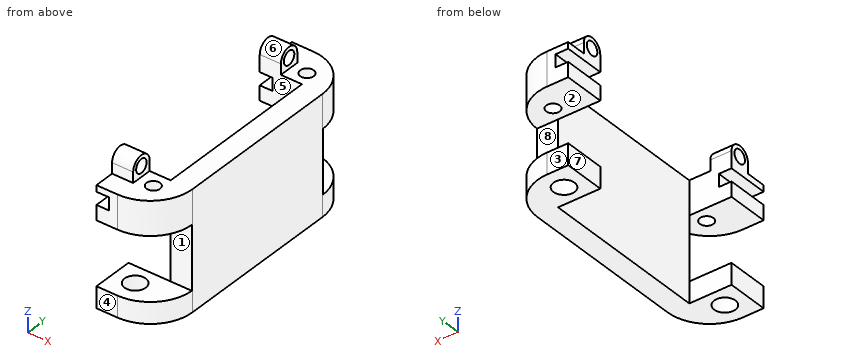
from build123d import *
from build123d.topology import SkipClean

# Parameters (mm, degrees)
BOSS_EXTRUDE1_DEPTH = 8
SKETCH2_W           = 20
SKETCH2_H           = 40
BOSS_EXTRUDE2_DEPTH = 5
SKETCH3_W           = 5
SKETCH3_H           = 5
BOSS_EXTRUDE3_DEPTH = 5
FILLET2_RADIUS      = 2.5
FILLET2_LENGTH      = 5
FILLET3_RADIUS      = 2.5
FILLET3_LENGTH      = 5
SKETCH6_R           = 1.6
CUT_EXTRUDE3_DEPTH  = 34.541019662
BOSS_EXTRUDE4_DEPTH = 5
BOSS_EXTRUDE5_DEPTH = 5
SKETCH11_W          = 15
SKETCH11_H          = 4.771622141
BOSS_EXTRUDE6_DEPTH = 8
FILLET4_R           = 10
FILLET5_START       = -21
FILLET5_DEPTH       = 30
SKETCH12_R          = 1.6
CUT_EXTRUDE4_DEPTH  = 10
SKETCH15_W          = 6
SKETCH15_H          = 3
CUT_EXTRUDE7_DEPTH  = 20
SKETCH17_W          = 6
SKETCH17_H          = 3
CUT_EXTRUDE8_DEPTH  = 20


with BuildPart() as part:
    # Sketch1 → Boss-Extrude1 (new body)
    with BuildSketch(Plane.XY):
        Polygon((-5, 25), (10, 25), (10, -25), (-5, -25), (-5, -20), (5, -20), (5, 20), (-5, 20), align=None)
    extrude(amount=BOSS_EXTRUDE1_DEPTH)

    # Sketch2 → Boss-Extrude2 (add)
    with BuildSketch(Plane(origin=(10, 0, 0), x_dir=(0, 0, -1), z_dir=(1, 0, 0))):
        with Locations((10, 0)):
            Rectangle(SKETCH2_W, SKETCH2_H)
    extrude(amount=-BOSS_EXTRUDE2_DEPTH)

    # Sketch3 → Boss-Extrude3 (add)
    with BuildSketch(Plane.XY.offset(8)):
        with Locations((-2.5, 22.5)):
            Rectangle(SKETCH3_W, SKETCH3_H)
        with Locations((-2.5, -22.5)):
            Rectangle(SKETCH3_W, SKETCH3_H)
    extrude(amount=BOSS_EXTRUDE3_DEPTH)

    # Fillet2: full round fillet: the end face becomes a half cylinder, R = half its width
    fillet2_face = Plane((-2.5, 22.5, 13), x_dir=(1, 0, 0), z_dir=(0, 0, 1))  # on the end face: x along it, z out of the body
    fillet2_slab = fillet2_face.offset(-FILLET2_RADIUS / 2) * Box(FILLET2_LENGTH, 2 * FILLET2_RADIUS, FILLET2_RADIUS, mode=Mode.PRIVATE)  # the body's end, R deep
    fillet2_round = Plane((-2.5, 22.5, 10.5), x_dir=(0, 0, 1), z_dir=(1, 0, 0)) * Cylinder(FILLET2_RADIUS, FILLET2_LENGTH, mode=Mode.PRIVATE)  # its axis R under the face
    add(fillet2_slab - fillet2_round, mode=Mode.SUBTRACT)

    # Fillet3: full round fillet: the end face becomes a half cylinder, R = half its width
    fillet3_face = Plane((-2.5, -22.5, 13), x_dir=(1, 0, 0), z_dir=(0, 0, 1))  # on the end face: x along it, z out of the body
    fillet3_slab = fillet3_face.offset(-FILLET3_RADIUS / 2) * Box(FILLET3_LENGTH, 2 * FILLET3_RADIUS, FILLET3_RADIUS, mode=Mode.PRIVATE)  # the body's end, R deep
    fillet3_round = Plane((-2.5, -22.5, 10.5), x_dir=(0, 0, 1), z_dir=(1, 0, 0)) * Cylinder(FILLET3_RADIUS, FILLET3_LENGTH, mode=Mode.PRIVATE)  # its axis R under the face
    add(fillet3_slab - fillet3_round, mode=Mode.SUBTRACT)

    # Sketch6 → Cut-Extrude3 (cut, through all)
    with BuildSketch(Plane(origin=(0, 0, 0), x_dir=(0, 0, -1), z_dir=(1, 0, 0))):
        with Locations((-10.5, 22.5)):
            Circle(SKETCH6_R)
        with Locations((-10.5, -22.5)):
            Circle(SKETCH6_R)
    extrude(amount=-CUT_EXTRUDE3_DEPTH, mode=Mode.SUBTRACT)

    # Sketch7 → Boss-Extrude4 (add)
    with BuildSketch(Plane(origin=(0, 0, -20), x_dir=(-1, 0, 0), z_dir=(0, 0, -1))):
        with BuildLine():
            Line((5, 27.3), (5, 20))
            Line((5, 20), (-5, 20))
            Line((-5, 20), (-10, 20))
            Line((-10, 20), (-10, 27.3))
            Line((-10, 27.3), (-1.58, 27.3))
            Line((-1.58, 27.3), (-1.58, 26.5))
            ThreePointArc((-1.58, 26.5), (-0.08, 22), (1.42, 26.5))
            Line((1.42, 26.5), (1.42, 27.3))
            Line((1.42, 27.3), (5, 27.3))
        make_face()
    boss_extrude4 = extrude(amount=-BOSS_EXTRUDE4_DEPTH)

    # Mirror3: Boss-Extrude4 across plane
    add(boss_extrude4.mirror(Plane.ZX))

    # Sketch10 → Boss-Extrude5 (add)
    with SkipClean():  # the faces are left unmerged after this step: merging them gives an invalid solid
        with BuildSketch(Plane(origin=(0, 0, -20), x_dir=(-1, 0, 0), z_dir=(0, 0, -1))):
            with BuildLine():
                Line((5, 29.771622141), (-10, 29.771622141))
                Line((-10, 29.771622141), (-10, 27.3))
                Line((-10, 27.3), (-1.58, 27.3))
                Line((-1.58, 27.3), (-1.58, 26.5))
                ThreePointArc((-1.58, 26.5), (-0.08, 27), (1.42, 26.5))
                Line((1.42, 26.5), (1.42, 27.3))
                Line((1.42, 27.3), (5, 27.3))
                Line((5, 27.3), (5, 29.771622141))
            make_face()
        boss_extrude5 = extrude(amount=-BOSS_EXTRUDE5_DEPTH)

    # Mirror4: Boss-Extrude5 across plane
    with SkipClean():  # the faces are left unmerged after this step: merging them gives an invalid solid
        add(boss_extrude5.mirror(Plane.ZX))

    # Sketch11 → Boss-Extrude6 (add)
    with SkipClean():  # the faces are left unmerged after this step: merging them gives an invalid solid
        with BuildSketch(Plane.XY.offset(8)):
            with Locations((2.5, 27.385811071)):
                Rectangle(SKETCH11_W, SKETCH11_H)
            with Locations((2.5, -27.385811071)):
                Rectangle(SKETCH11_W, SKETCH11_H)
        extrude(amount=-BOSS_EXTRUDE6_DEPTH)

    # Fillet4
    # the kernel refuses this fillet: 10 mm, written as the material it takes off along each edge
    with BuildSketch(Plane(origin=(10, 29.771622141, 33), x_dir=(0, -1, 0), z_dir=(0, 0, -1))) as fillet4_piece_1:
        with BuildLine():
            CenterArc((FILLET4_R, FILLET4_R), FILLET4_R, 180, 90)
            Line((0, FILLET4_R), (0, 0))
            Line((0, 0), (FILLET4_R, 0))
        make_face()
    extrude(amount=58, mode=Mode.SUBTRACT)

    # Fillet5: read off the stored shape, not the designer's step
    # Fillet5 outline → Fillet5 (cut)
    with BuildSketch(Plane.XY.offset(FILLET5_START)):
        with BuildLine():
            Line((10, -29.771622141), (10, -19.771622141))
            ThreePointArc((10, -19.771622141), (7.071067812, -26.842689953), (0, -29.771622141))
            Line((0, -29.771622141), (10, -29.771622141))
        make_face()
    extrude(amount=FILLET5_DEPTH, mode=Mode.SUBTRACT)

    # Sketch12 → Cut-Extrude4 (cut)
    with BuildSketch(Plane.XY.offset(8)):
        with Locations((3.535533906, 23.421344977)):
            Circle(SKETCH12_R)
        with Locations((3.535533906, -23.421344977)):
            Circle(SKETCH12_R)
    extrude(amount=-CUT_EXTRUDE4_DEPTH, mode=Mode.SUBTRACT)

    # Sketch15 → Cut-Extrude7 (cut)
    with BuildSketch(Plane.XZ.offset(29.771622141)):
        with Locations((-5, 5)):
            Rectangle(SKETCH15_W, SKETCH15_H)
    extrude(amount=-CUT_EXTRUDE7_DEPTH, mode=Mode.SUBTRACT)

    # Sketch17 → Cut-Extrude8 (cut)
    with BuildSketch(Plane(origin=(0, 29.771622141, 0), x_dir=(1, 0, 0), z_dir=(0, 1, 0))):
        with Locations((-5, -5)):
            Rectangle(SKETCH17_W, SKETCH17_H)
    extrude(amount=-CUT_EXTRUDE8_DEPTH, mode=Mode.SUBTRACT)


solid = part.part
CAD build for the part. Positions are in the model's coordinates, mm. Face numbers are marked on the shaded views. A direction names the side the tool comes from. Round coordinates to 2 decimals unless told otherwise and drop trailing zeros. Write each loop counter-clockwise with the first axis right and the second up, starting at its lowest first coordinate (ties: lowest second). Pieces come first, ordered by that corner, then holes. Notation, with made-up numbers: M 11,-33 L 56,-33 A16 cw 56,-26 Z; hole C -2,89 d5. An arc over 180 degrees is marked long. Put each result on its own line as item: value. Start each with the question number.
1) Pin check, flat tips, straight feed: pin 1 Ø2.5 at (x, y) = (3.54, 23.42) entering from +Z; pin 2 Ø5.5 at (y, z) = (-22.5, 11) entering from +X; pin 3 Ø1.5 at (x, z) = (7.5, -11) entering from +Y. Stop position of each tip, or through.
2) Saw through at A-A, the plane x = -3.75. Count the separate pieces of the cut face and the enclosed holes in it, and give its area (3 significant figures).
3) Saw through at C-C, the plane z = 4.5. Write the cut outline in (x, y).
4) Saw through at D-D, the plane z = -11.5. Write the cut outline in (x, y).
5) Saw through at B-B, the plane x = 0.75. Write the cut outline in (y, z).
6) Drill centre lines: probe 1 along Y at (x, z) = (0.08, -18.1); probe 2 along Z at (x, y) = (8.5, -22); probe 3 along Y at (x, z) = (-3.65, 10.5). Where is each one in solid material? Low to high. Write a range as [from, to].
7) 3-axis set-ups, long thin cutter, end or side, ignore diameter. For the marked faces 1, 2, 3, 4 and 5: which of +Z, -Z, +X, -X, +Y, -Y reach the whole face in a straight line?
8) Pull direction Z, two halves, no side cores. Call the marked faces 6, 7 and 8: pulls with the +Z half, pulls with the -Z half, needs draft (parallel to the pull), parting line crosses it, or undercut.
Resolved:
1. pin 1: z = -15
1. pin 2: x = 0
1. pin 3: y = 20
2. separate pieces: 6
2. enclosed holes: 2
2. area: 224 mm²
3. outline: M -2,-29.77 L 0,-29.77 A10 ccw 10,-19.77 L 10,19.77 A10 ccw 0,29.77 L -2,29.77 L -2,20 L 5,20 L 5,-20 L -2,-20 Z; hole C 3.54,-23.42 d3.2; hole C 3.54,23.42 d3.2
4. outline: M 5,-20 L 10,-20 A10 ccw 10,-19.77 L 10,19.77 A10 ccw 10,20 L 5,20 Z
5. outline: M -29.74,-20 L -26.91,-20 L -26.91,-15 L -29.74,-15 Z; M -29.74,0 L -20,0 L -20,8 L -29.74,8 Z; M -22.09,-20 L -20,-20 L -20,-15 L -22.09,-15 Z; M 20,-20 L 22.09,-20 L 22.09,-15 L 20,-15 Z; M 20,0 L 29.74,0 L 29.74,8 L 20,8 Z; M 26.91,-20 L 29.74,-20 L 29.74,-15 L 26.91,-15 Z
6. probe 1: [-29.77, -27], [-22, -20], [20, 22], [27, 29.77]
6. probe 2: [-20, -15], [0, 8]
6. probe 3: [-25, -24.1], [-20.9, -20], [20, 20.9], [24.1, 25]
7. face 1: +X, -X, -Y
7. face 2: +X, -X, +Y
7. face 3: +Z, -Z, +X, -X, +Y
7. face 4: +Z, -Z, +X, -X, -Y
7. face 5: +Z, -Z, -X
8. face 6: pulls with the +Z half
8. face 7: needs draft
8. face 8: undercut
